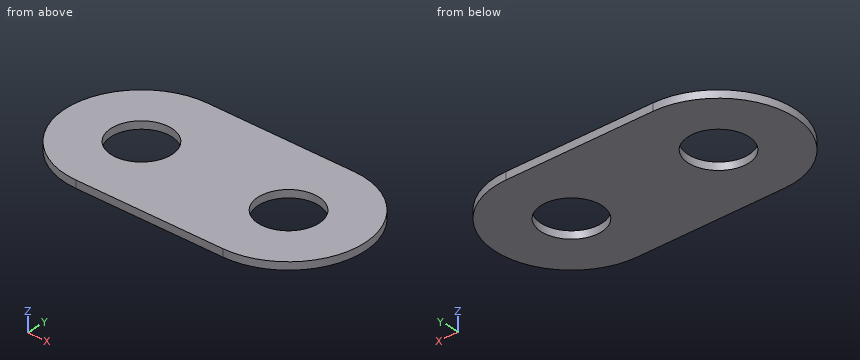
Autodesk Inventor part; units mm, degrees
ref_plane "YZ Plane" through (0, 0, 0) normal (1, 0, 0) x (0, 1, 0)
ref_plane "XZ Plane" through (0, 0, 0) normal (0, 1, 0) x (-1, 0, 0)
ref_plane "XY Plane" through (0, 0, 0) normal (0, 0, 1) x (1, 0, 0)
sketch "Náčrt1" plane through (0, 0, 0) normal (0, 0, 1) x (1, 0, 0)
  line L0 (-5, 0) -> (5, 0) construction
  line L1 (-5, -5) -> (5, -5)
  line L2 (5, 5) -> (-5, 5)
  arc A0 (-5, 5) -> (-5, -5) centre (-5, 0) ccw
  arc A1 (5, -5) -> (5, 5) centre (5, 0) ccw
  point P0 (0, 0)
  point P1 (10, 0)
  dimension "d0" = 10
  dimension "d1" = 5
extrude "Vysunutí1" add sketch "Náčrt1" along normal blind 0.5
sketch "Náčrt2" plane through (0, 0, 0) normal (0, 0, -1) x (-1, 0, 0)
  arc A0 (5, -5) -> (5, 5) centre (5, 0) ccw
  circle A1 centre (5, 0) radius 2
  point P0 (0, 0)
  dimension "d4" = 4
extrude "Vysunutí2" cut sketch "Náčrt2" against normal through all
pattern_linear "Obdélníkové pole1" count 7 spacing 10 along (1, 0, 0) of "Vysunutí2"
properties part number "1002"
For this review, take the finished solid that the model builds, in its own axes (mm). Round coordinates to 2 decimals unless told otherwise and drop trailing zeros. Loops run counter-clockwise (first coordinate to the right, second up) from the corner with the lowest first, then second, coordinate; pieces in that order, holes last. Notation, with made-up numbers: (-21, 75) - (-14, 75) arc R26 ccw to (-14, 90) - close; hole circle Ø1 at (-24.5, -29.5). An arc over 180 degrees is marked (long way). One line per question, with ' | ' between items.
Q1. For line 1 along Y through (x, z) = (-5, 0.4); line 2 along Y through (x, z) = (9, 0.2); line 3 along X through (y, z) = (1.75, 0.35), list the stretches that pass through material, from the lowest coordinate up. Write a range as [from, to].
Taken from the geometry:
line 1: y = [-5, -2], [2, 5] | line 2: y = [-3, 3] | line 3: x = [-9.68, -5.97], [-4.03, 4.03], [5.97, 9.68]
Q2. Take a section at D-D (y = -3). Give the boundary of the cut face in (x, z), and give its area (3 significant figures).
Taken from the geometry:
outline: (-9, 0) - (9, 0) - (9, 0.5) - (-9, 0.5) - close | area: 9.00 mm²
Q3. For pin 1 (2.5 mm diameter, centred on x = 5, y = 0, fed in from +Z), flat-tipped, find the tip position at first contact; note if it passes through.
Taken from the geometry:
pin 1: passes through
Q4. Take a section at B-B (z = 0.3). Give the boundary of the cut face in (x, y), and give its area (3 significant figures).
Taken from the geometry:
outline: (-5, -5) - (5, -5) arc R5 ccw to (5, 5) - (-5, 5) arc R5 ccw to start; hole circle Ø4 at (-5, 0); hole circle Ø4 at (5, 0) | area: 153 mm²
Q5. Take a section at A-A (y = 0). Give the boundary of the cut face in (x, z).
Taken from the geometry:
outline: (-10, 0) - (-7, 0) - (-7, 0.5) - (-10, 0.5) - close; (-3, 0) - (3, 0) - (3, 0.5) - (-3, 0.5) - close; (7, 0) - (10, 0) - (10, 0.5) - (7, 0.5) - close
Q6. Take a section at C-C (x = 5.5). Give the boundary of the cut face in (y, z), and give its area (3 significant figures).
Taken from the geometry:
outline: (-4.97, 0) - (-1.94, 0) - (-1.94, 0.5) - (-4.97, 0.5) - close; (1.94, 0) - (4.97, 0) - (4.97, 0.5) - (1.94, 0.5) - close | area: 3.04 mm²
